```python
from build123d import *

# Parameters (mm, degrees)
EXTRUDE_1_DEPTH = 2.9
SKETCH_2_W      = 0.293894488
SKETCH_2_H      = 0.44460961
EXTRUDE_2_DEPTH = 5


with BuildPart() as part:
    # Эскиз1 → Бобышка-Вытянуть1 (new body)
    with BuildSketch(Plane.XY):
        Polygon((-392.814753218, 89.720587497), (-392.314753218, 90.920587497), (-390.314753218, 90.920587497), (-389.814753218, 89.720587497), (-389.814753218, 88.120587497), (-390.314753218, 86.920587497), (-392.314753218, 86.920587497), (-392.814753218, 88.120587497), align=None)
    extrude(amount=EXTRUDE_1_DEPTH)

    # Эскиз2 → Бобышка-Вытянуть2 (add)
    with BuildSketch(Plane.XY.offset(2.9)):
        with Locations((-390.83341038, 90.168528042)):
            Rectangle(SKETCH_2_W, SKETCH_2_H)
        with Locations((-391.83341038, 90.168528042)):
            Rectangle(SKETCH_2_W, SKETCH_2_H)
        with Locations((-390.83341038, 88.968528042)):
            Rectangle(SKETCH_2_W, SKETCH_2_H)
        with Locations((-390.83341038, 87.768528042)):
            Rectangle(SKETCH_2_W, SKETCH_2_H)
        with Locations((-391.83341038, 88.968528042)):
            Rectangle(SKETCH_2_W, SKETCH_2_H)
        with Locations((-391.83341038, 87.768528042)):
            Rectangle(SKETCH_2_W, SKETCH_2_H)
    extrude(amount=EXTRUDE_2_DEPTH)


solid = part.part
```
Model file for the job. Use its own axes, mm. Give positions to 0.01 mm unless a question says otherwise; leave off trailing zeros. Write each loop counter-clockwise with the first axis right and the second up, starting at its lowest first coordinate (ties: lowest second). Pieces come first, ordered by that corner, then holes. Notation, with made-up numbers: (-16, 2) -> (26, 2) arc R21 cw to (26, 30) -> close; hole circle Ø1 at (88.5, 75). An arc over 180 degrees is marked (long way). Use CSV: the item, a comma, the result in double quotes. Start each with the question number.
1) Cut at D-D on z = 2.5. List the corners of the cut face in (x, y), plus the area to 3 significant figures.
2) Drill centre lines: L1, parallel to X at y = 87.7, z = 4.75; L2, parallel to Z at x = -391.55, y = 89.15; L3, parallel to X at y = 87.5, z = 0.75. Where is each one in solid material? Low to high.
3) Cut at A-A on z = 5.5. List the corners of the cut face in (x, y), plus the area to 3 significant figures.
4) Pin check, flat tips, straight feed: P1, Ø1, axis at y = 90, z = 7, coming from the +X side; P2, Ø1.5, axis at x = -390.5, z = 5, coming from the -Y side. Stop position of each tip, or through.
5) Cut at B-B on x = -390.8. List the corners of the cut face in (y, z).
6) Cut at C-C on y = 89. List the corners of the cut face in (x, z), plus the area to 3 significant figures.
Final values:
1,outline,"(-392.81, 88.12) -> (-392.31, 86.92) -> (-390.31, 86.92) -> (-389.81, 88.12) -> (-389.81, 89.72) -> (-390.31, 90.92) -> (-392.31, 90.92) -> (-392.81, 89.72) -> close"
1,area,"10.8 mm2"
2,L1,"x = -391.98 to -391.69, -390.98 to -390.69"
2,L2,"z = 0 to 2.9"
2,L3,"x = -392.56 to -390.07"
3,outline,"(-391.98, 87.55) -> (-391.69, 87.55) -> (-391.69, 87.99) -> (-391.98, 87.99) -> close; (-391.98, 88.75) -> (-391.69, 88.75) -> (-391.69, 89.19) -> (-391.98, 89.19) -> close; (-391.98, 89.95) -> (-391.69, 89.95) -> (-391.69, 90.39) -> (-391.98, 90.39) -> close; (-390.98, 87.55) -> (-390.69, 87.55) -> (-390.69, 87.99) -> (-390.98, 87.99) -> close; (-390.98, 88.75) -> (-390.69, 88.75) -> (-390.69, 89.19) -> (-390.98, 89.19) -> close; (-390.98, 89.95) -> (-390.69, 89.95) -> (-390.69, 90.39) -> (-390.98, 90.39) -> close"
3,area,"0.784 mm2"
4,P1,"stops at x = -390.69"
4,P2,"stops at y = 87.55"
5,outline,"(86.92, 0) -> (90.92, 0) -> (90.92, 2.9) -> (90.39, 2.9) -> (90.39, 7.9) -> (89.95, 7.9) -> (89.95, 2.9) -> (89.19, 2.9) -> (89.19, 7.9) -> (88.75, 7.9) -> (88.75, 2.9) -> (87.99, 2.9) -> (87.99, 7.9) -> (87.55, 7.9) -> (87.55, 2.9) -> (86.92, 2.9) -> close"
6,outline,"(-392.81, 0) -> (-389.81, 0) -> (-389.81, 2.9) -> (-390.69, 2.9) -> (-390.69, 7.9) -> (-390.98, 7.9) -> (-390.98, 2.9) -> (-391.69, 2.9) -> (-391.69, 7.9) -> (-391.98, 7.9) -> (-391.98, 2.9) -> (-392.81, 2.9) -> close"
6,area,"11.6 mm2"
